```python
from build123d import *

# Parameters (mm, degrees)
F0_W        = 49
F0_H        = 19
F1_DEPTH    = 20
F2_R        = 4.5
F3_DEPTH    = 1.5
F4_DEPTH    = 19
F5_T        = 0.5
F5_T3_DEPTH = 19
F5_T5_DEPTH = 19


# Not quite as in the source:
# - a shell that OpenCascade refuses in one call is made with other operations: the cavity is built on its own and cut out


with BuildPart() as f1:
    # F0 (on Front) → F1 (new body, symmetric)
    with BuildSketch(Plane.XZ):
        with Locations((1.5, 9.5)):
            Rectangle(F0_W, F0_H)
    extrude(amount=F1_DEPTH, both=True)

    # F2 (on face) → F3 (join)
    with BuildSketch(Plane.YZ.offset(26)):
        Polygon((-9, 19), (-9, 1), (0, 1), (9, 1), (9, 19), (0, 19), align=None)
        with Locations((0, 10)):
            Circle(F2_R, mode=Mode.SUBTRACT)
    extrude(amount=F3_DEPTH)

    # F4 (add): a face of the model
    f4_faces = [f1.faces().sort_by_distance(p)[0] for p in [
        (26, 0, 10),
    ]]
    extrude(f4_faces, amount=F4_DEPTH)

    # F5: shell of thickness 0.5, made by hand


with BuildPart() as f5_core1:
    # F5_t2: copy of F1
    add(f1.part)

    # the walls: a layer under each face that stays
    f5_faces = [f5_core1.faces().sort_by_distance(p)[0] for p in [
        (2.25, 0, 19),
        (1.5, 20, 9.5),
        (-23, 0, 9.5),
        (1.5, -20, 9.5),
        (26, 13.3333333333, 3.1666666667),
        (26.75, -9, 10),
        (27.5, -6, 4),
        (26.75, 9, 10),
        (1.5, 0, 0),
        (26.75, 0, 1),
        (36.25, -4.5, 10),
    ]]
    thicken(f5_faces, amount=-F5_T, mode=Mode.SUBTRACT)

    # F5_s4 → F5_t3 (cut)
    with BuildSketch(Plane.XY.offset(0.5)):
        Polygon((26.005, -9.005), (25.5, -9), (25.5, -8.5), (26, -8.5), align=None)
        Polygon((26.005, 9.005), (25.5, 9), (25.5, 8.5), (26, 8.5), align=None)
    extrude(amount=F5_T3_DEPTH, mode=Mode.SUBTRACT)

    # F5_s6 → F5_t5 (cut)
    with BuildSketch(Plane.XZ.offset(-9.5)):
        Polygon((26.005, 0.995), (25.5, 1), (25.5, 1.5), (26, 1.5), align=None)
    extrude(amount=F5_T5_DEPTH, mode=Mode.SUBTRACT)

    # F5_s7 → F5_t8 (revolve, cut)
    with BuildSketch(Plane.XY.offset(10)):
        Polygon((27.505, 4.505), (27, 4.5), (27, 4), (27.5, 4), align=None)
    revolve(axis=Axis((27.5, 0, 10), (1, 0, 0)), mode=Mode.SUBTRACT)


with BuildPart() as f1_1:
    add(f1.part)

    # what is left inside the walls is the cavity
    f5_cavity = [f5_core1.part.solids().sort_by_distance(p)[0] for p in [
        (2.25, 6.5, 18.495),
    ]]
    add(f5_cavity, mode=Mode.SUBTRACT)


solid = f1_1.part
```
Geometry: final body of the model. Coordinates: model frame, mm. A direction names the side the tool comes from. Round coordinates to 2 decimals unless told otherwise and drop trailing zeros. Order: outer loops, then holes, each group sorted by start corner. A loop starts at its lowest first (then second) coordinate and runs counter-clockwise, first axis right, second up. Notation, with made-up numbers: (18.5, -36) -> (63.5, -36) arc R28 ccw to (63.5, -6) -> close; hole circle Ø8 at (-7, 5). An arc over 180 degrees is marked (long way). Use CSV: the item, a comma, the result in double quotes. Start each with the question number.
1) Material intervals for line 1 along Z through (x, y) = (-12, 18.5); line 2 along Y through (x, z) = (14.5, 16.25); line 3 along X through (y, z) = (14, 10.5), sorted ascending. Write a range as from..to.
2) Section C-C (z = 15.25). Return the cut outline in (x, y).
3) Section A-A (y = -10). Return the cut outline in (x, z).
4) Section B-B (x = 1). Return the cut outline in (y, z), and give its area (3 significant figures).
5) Set-up query: faces 5 (the face through (27, 9, 10)), 6 (the face through (27, 4, 12)), 7 (the face through (27, -9, 10)), 8 (the face through (36.13, -0.59, 14.46)), 9 (the face through (27, 0, 1)). Return all of +Z, -Z, +X, -X, +Y, -Y with unobstructed straight access to the full face (end or side cutting, diameter ignored); none if empty.
6) First-contact query: pin 1 Ø3 at (y, z) = (7, 5) entering from +X; pin 2 Ø0.8 at (x, z) = (26.5, 13.5) entering from -Y; pin 3 Ø0.8 at (x, y) = (26.5, 1.5) entering from -Z. Flat tips, straight axial feed; report the tip coordinate or a pass-through.
7) Draft query along Z for faces 1 (the face through (27.5, -4, 14)), 2 (the face through (2, 0, 18.5)), 3 (the face through (2, 0, 19)), 4 (the face through (-22.5, 0, 9)). Return one class per face: +Z half, -Z half, draft (parallel to the pull), parting line (faces both ways), or undercut.
8) Section D-D (z = 10). Return the cut outline in (x, y).
Returned:
1,line 1,"z = 0..0.5, 18.5..19"
1,line 2,"y = -20..-19.5, 19.5..20"
1,line 3,"x = -23..-22.5, 25.5..26"
2,outline,"(-23, -20) -> (26, -20) -> (26, -9) -> (27.5, -9) -> (27.5, 9) -> (26, 9) -> (26, 20) -> (-23, 20) -> close; hole (-22.5, -19.5) -> (25.5, -19.5) -> (25.5, -8.5) -> (27, -8.5) -> (27, 8.5) -> (25.5, 8.5) -> (25.5, 19.5) -> (-22.5, 19.5) -> close"
3,outline,"(-23, 0) -> (26, 0) -> (26, 19) -> (-23, 19) -> close; hole (-22.5, 0.5) -> (25.5, 0.5) -> (25.5, 18.5) -> (-22.5, 18.5) -> close"
4,outline,"(-20, 0) -> (20, 0) -> (20, 19) -> (-20, 19) -> close; hole (-19.5, 0.5) -> (19.5, 0.5) -> (19.5, 18.5) -> (-19.5, 18.5) -> close"
4,area,"58.0 mm²"
5,face 5,"+Z, -Z, +X, +Y"
5,face 6,"none"
5,face 7,"+Z, -Z, +X, -Y"
5,face 8,"+X"
5,face 9,"-Z, +X, +Y, -Y"
6,pin 1,"stops at x = 27.5"
6,pin 2,"stops at y = -9"
6,pin 3,"stops at z = 1"
7,face 1,"draft"
7,face 2,"undercut"
7,face 3,"+Z half"
7,face 4,"undercut"
8,outline,"(-23, -20) -> (26, -20) -> (26, -9) -> (27.5, -9) -> (27.5, -4.5) -> (45, -4.5) -> (45, -4) -> (27, -4) -> (27, -8.5) -> (25.5, -8.5) -> (25.5, -19.5) -> (-22.5, -19.5) -> (-22.5, 19.5) -> (25.5, 19.5) -> (25.5, 8.5) -> (27, 8.5) -> (27, 4) -> (45, 4) -> (45, 4.5) -> (27.5, 4.5) -> (27.5, 9) -> (26, 9) -> (26, 20) -> (-23, 20) -> close"
